```python
from build123d import *

# Parameters (mm, degrees)
BASE_DEPTH             = 25
ESQUISSE2_W            = 3.051401781
ESQUISSE2_H            = 3.671186171
VIDE_BASE_DEPTH        = 25
CONG_2_R               = 2
VIDE_BASE_2_DEPTH      = 14
VIDE_BASE_2_DEPTH_BACK = 14
AXE_ROUE_DEPTH         = 11
AXE_ROUE_DEPTH_BACK    = 11
ESQUISSE7_R            = 3
CONGE_VIS_1_R          = 1
CONGE_VIS_2_R          = 1


with BuildPart() as part:
    # Esquisse1 → BASE (new body)
    with BuildSketch(Plane(origin=(0, 0, 0), x_dir=(0, 0, -1), z_dir=(1, 0, 0))):
        with BuildLine():
            Line((5.371432156, 1.182250648), (2, 16.5))
            Line((2, 16.5), (-27, 16.5))
            Line((-27, 16.5), (-27, 12))
            Line((-27, 12), (-24.881319015, 12))
            ThreePointArc((-24.881319015, 12), (-21.262987094, 11.322428552), (-18.134990853, 9.381534822))
            Line((-18.134990853, 9.381534822), (-4.641317523, -2.950961141))
            ThreePointArc((-4.641317523, -2.950961141), (2.098601145, -5.083883676), (5.371432156, 1.182250648))
        make_face()
    extrude(amount=BASE_DEPTH)

    # Esquisse2 → VIDE BASE (cut)
    with BuildSketch(Plane(origin=(0, 16.5, 0), x_dir=(1, 0, 0), z_dir=(0, 1, 0))):
        with BuildLine():
            Line((25, 2), (21.948598219, 2))
            add(Edge.make_bspline(
                [(23.267838517, -8.151484137), (21.529216313, -3.190142242), (21.948598219, 2)],
                knots=[0, 0, 0, 1, 1, 1], degree=2))
            ThreePointArc((23.267838517, -8.151484137), (24.559186985, -11.209709851), (25, -14.5))
            Line((25, -14.5), (25, 2))
        make_face()
        with Locations((23.47429911, 3.835593086)):
            Rectangle(ESQUISSE2_W, ESQUISSE2_H)
        with Locations((1.525700891, 3.835593086)):
            Rectangle(ESQUISSE2_W, ESQUISSE2_H)
        with BuildLine():
            add(Edge.make_bspline(
                [(1.732161483, -8.151484137), (3.470783687, -3.190142242), (3.051401781, 2)],
                knots=[0, 0, 0, 1, 1, 1], degree=2))
            Line((3.051401781, 2), (0, 2))
            Line((0, 2), (0, -14.49999997))
            ThreePointArc((0, -14.49999997), (0.440813019, -11.209709836), (1.732161483, -8.151484137))
        make_face()
        with BuildLine():
            Line((0, -27), (12.5, -27))
            ThreePointArc((12.5, -27), (3.661165225, -23.338834754), (0, -14.49999997))
            Line((0, -14.49999997), (0, -27))
        make_face()
        with BuildLine():
            Line((25, -27), (25, -14.5))
            ThreePointArc((25, -14.5), (21.338834765, -23.338834765), (12.5, -27))
            Line((12.5, -27), (25, -27))
        make_face()
    extrude(amount=-VIDE_BASE_DEPTH, mode=Mode.SUBTRACT)

    # Esquisse4 → VIS (revolve)
    with BuildSketch(Plane.ZY.offset(-12.5), mode=Mode.PRIVATE) as vis_sk:
        Polygon((14.5, 16.5), (14.5, 33.5), (17.5, 33.5), (17.5, 23.5), (19.5, 23.5), (19.5, 18.5), (26.5, 18.5), (26.5, 16.5), align=None)
    revolve(vis_sk.sketch.rotate(Axis((12.5, 16.5, 14.5), (0, 1, 0)), 180), axis=Axis((12.5, 16.5, 14.5), (0, 1, 0)))

    # Congé2
    cong_2_edges = [part.edges().sort_by_distance(p)[0] for p in [
        (12.5, 18.5, 26.5),
    ]]
    fillet(cong_2_edges, radius=CONG_2_R - 0.0001)  # a hair under: the kernel refuses the full size

    # Esquisse6 → VIDE BASE 2 (cut, two sides: drawn at the far end of the back side and taken through both)
    with BuildSketch(Plane(origin=(0, 0, 0), x_dir=(1, 0, 0), z_dir=(0, 1, 0)).offset(-VIDE_BASE_2_DEPTH_BACK)):
        with BuildLine():
            Line((4.051401781, 5.5), (4.051401781, -5.609523223))
            ThreePointArc((4.051401781, -5.609523223), (12.5, -25.384659014), (20.948598219, -5.609523223))
            Line((20.948598219, -5.609523223), (20.948598219, 5.5))
            Line((20.948598219, 5.5), (4.051401781, 5.5))
        make_face()
    extrude(amount=VIDE_BASE_2_DEPTH + VIDE_BASE_2_DEPTH_BACK, mode=Mode.SUBTRACT)

    # Esquisse7 → AXE ROUE (add, two sides: drawn at the far end of the back side and taken through both)
    with BuildSketch(Plane.ZY.offset(-12.5).offset(-AXE_ROUE_DEPTH_BACK)):
        Circle(ESQUISSE7_R)
    extrude(amount=AXE_ROUE_DEPTH + AXE_ROUE_DEPTH_BACK)

    # CONGE VIS 1
    conge_vis_1_edges = [part.edges().sort_by_distance(p)[0] for p in [
        (23.5, 0, -3),
    ]]
    fillet(conge_vis_1_edges, radius=CONGE_VIS_1_R)

    # CONGE VIS 2
    conge_vis_2_edges = [part.edges().sort_by_distance(p)[0] for p in [
        (1.5, 0, -3),
    ]]
    fillet(conge_vis_2_edges, radius=CONGE_VIS_2_R)

    # Esquisse9 → ROUE (revolve)
    with BuildSketch(Plane(origin=(0, 0, 0), x_dir=(1, 0, 0), z_dir=(0, 1, 0))):
        Polygon((18.5, -4), (18.5, -3), (6.5, -3), (6.5, -4), (11.5, -4), (11.5, -12), (6.5, -12), (6.5, -13), (18.5, -13), (18.5, -12), (13.5, -12), (13.5, -4), align=None)
    revolve(axis=Axis((7.793426375, 0, 0), (1, 0, 0)))


solid = part.part
```
Design review of the part built by this model. Coordinates are the model's own, in mm. A direction names the side the tool comes from. Round coordinates to 2 decimals unless told otherwise and drop trailing zeros. Order: outer loops, then holes, each group sorted by start corner. A loop starts at its lowest first (then second) coordinate and runs counter-clockwise, first axis right, second up. Notation, with made-up numbers: M 25.5,-24 L 41.5,-24 A24 ccw 41.5,-8 Z; hole C 69,36 d7. An arc over 180 degrees is marked long. Put each result on its own line as item: value.
Q1. Consider section C-C (z = -8.5). State the section outline as (x, y) points.
Reported:
outline: M 6.5,-9.84 L 18.5,-9.84 L 18.5,-8.47 L 13.5,-8.47 L 13.5,8.47 L 18.5,8.47 L 18.5,9.84 L 6.5,9.84 L 6.5,8.47 L 11.5,8.47 L 11.5,-8.47 L 6.5,-8.47 Z
Q2. To check wall thickness, follow line 1 (Y direction, x = 9.95, z = 0); line 2 (Z direction, x = 17.05, y = 0); line 3 (X direction, y = 2.5, z = -5). State the ranges of each line that lie inside material, in increasing order.
Reported:
line 1: -13 to -12, -4 to 4, 12 to 13, 14 to 16.5
line 2: -13 to -12, -4 to 4, 12 to 13
line 3: 3.05 to 4.05, 11.5 to 13.5, 20.95 to 21.95
Q3. Draft analysis for pull direction Z (two halves, no side actions). For faces 6 (the face through (9.035, 3.905, -0.867)), 7 (the face through (3.511, -5.124, -1.999)), 8 (the face through (18.5, 9, 9)), state which applies: released by +Z, released by -Z, zero draft, split by the parting line, or undercut.
Reported:
face 6: undercut
face 7: split by the parting line
face 8: zero draft
Q4. Consider section B-B (y = -6.5). State the section outline as (x, z) points.
Reported:
outline: M 6.5,-11.26 L 18.5,-11.26 L 18.5,-10.09 L 13.5,-10.09 L 13.5,10.09 L 18.5,10.09 L 18.5,11.26 L 6.5,11.26 L 6.5,10.09 L 11.5,10.09 L 11.5,-10.09 L 6.5,-10.09 Z
Q5. Machinability: for faces 1 (the face through (7.543, 20.965, 15.151)), 2 (the face through (22.918, 9.425, 8.384)), 3 (the face through (13.5, -3, -3)), 4 (the face through (23.5, 0, 0)), 5 (the face through (13.156, 14.479, -2.445)), which of the approach directions +Z, -Z, +X, -X, +Y, -Y give a long, thin tool a straight path to every point of the face, cutting with its end or side? Answer none if there is none.
Reported:
face 1: +Y
face 2: -Y
face 3: none
face 4: -Z, +X, +Y, -Y
face 5: -Z, +Y
Q6. Consider section A-A (x = 10.75). State how many separate pieces and enclosed holes the cut face has, and give its area (3 significant figures).
Reported:
separate pieces: 3
enclosed holes: 1
area: 346 mm²
Q7. Insertion check: pin 1 Ø10 at (y, z) = (7.5, 2.5) entering from +X; pin 2 Ø19 at (y, z) = (0, 0) entering from +X; pin 3 Ø6.5 at (y, z) = (2, -0.5) entering from +X. Each pin has a flat end and moves straight along its axis. Give the tip position at first contact, or say it passes through.
Reported:
pin 1: x = 23.05
pin 2: x = 23.91
pin 3: x = 23.5
